Verification items for this drawing (mm, ordinates from the low corner). Round coordinates to 2 decimals unless told otherwise and drop trailing zeros. Order: outer loops, then holes, each group sorted by start corner. A loop starts at its lowest first (then second) coordinate and runs counter-clockwise, first axis right, second up. Notation, with made-up numbers: (85.5, -18) -> (129.5, -18) arc R33 ccw to (129.5, 17) -> close; hole circle Ø11 at (52.25, 16.5). An arc over 180 degrees is marked (long way). Put each result on its own line as item: value.
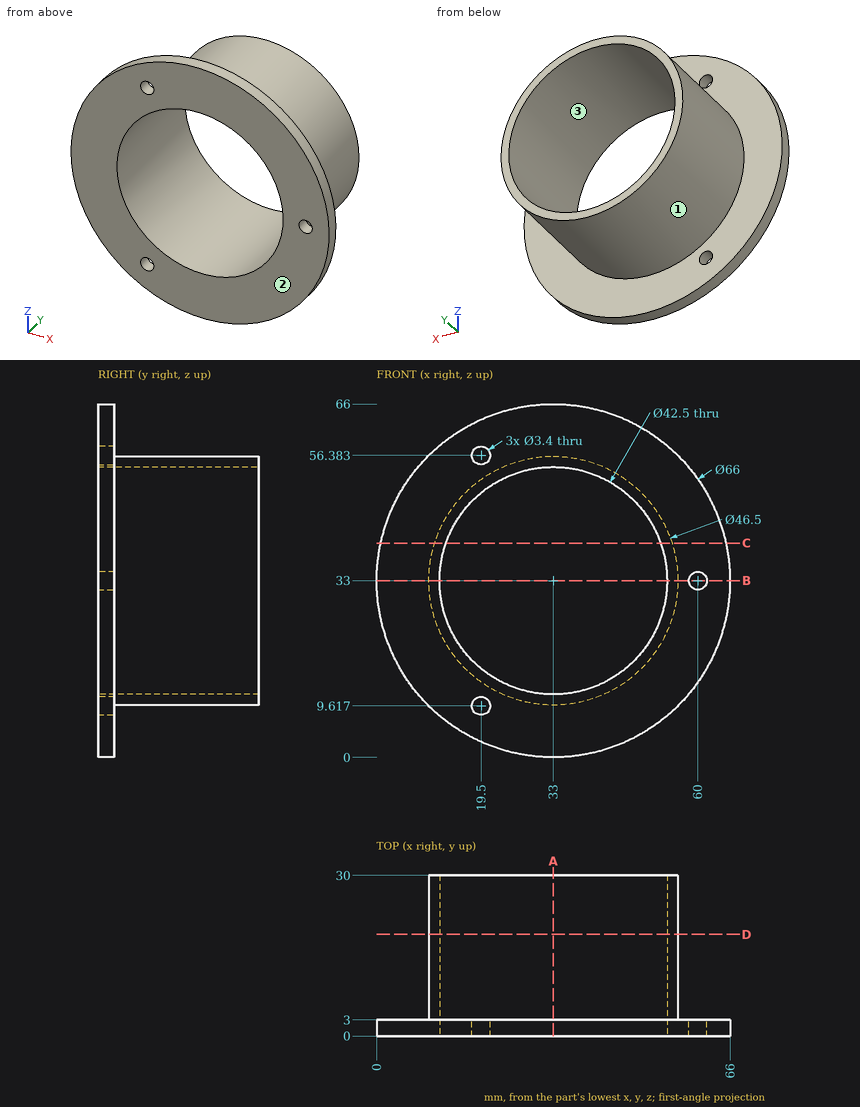
Item 1: Section check D-D on y = 19. Record the boundary of the cut face in (x, z).
Check sheet entries:
outline: circle Ø46.5 at (33, 33); hole circle Ø42.5 at (33, 33)
Item 2: Section check C-C on z = 40. Record the boundary of the cut face in (x, y), then the cut area to 3 significant figures.
Check sheet entries:
outline: (0.75, 0) -> (12.94, 0) -> (12.94, 30) -> (10.83, 30) -> (10.83, 3) -> (0.75, 3) -> close; (53.06, 0) -> (65.25, 0) -> (65.25, 3) -> (55.17, 3) -> (55.17, 30) -> (53.06, 30) -> close
area: 187 mm^2
Item 3: Section check B-B on z = 33. Record the boundary of the cut face in (x, y), then the cut area to 3 significant figures.
Check sheet entries:
outline: (0, 0) -> (11.75, 0) -> (11.75, 30) -> (9.75, 30) -> (9.75, 3) -> (0, 3) -> close; (54.25, 0) -> (58.3, 0) -> (58.3, 3) -> (56.25, 3) -> (56.25, 30) -> (54.25, 30) -> close; (61.7, 0) -> (66, 0) -> (66, 3) -> (61.7, 3) -> close
area: 168 mm^2
Item 4: Section check A-A on x = 33. Record the boundary of the cut face in (y, z).
Check sheet entries:
outline: (0, 0) -> (3, 0) -> (3, 9.75) -> (30, 9.75) -> (30, 11.75) -> (0, 11.75) -> close; (0, 54.25) -> (30, 54.25) -> (30, 56.25) -> (3, 56.25) -> (3, 66) -> (0, 66) -> close
Item 5: Release check for a two-part mould opening along Z. For the marked faces 1, 2 and 3 record: +Z half, -Z half, draft (parallel to the pull), parting line (faces both ways), or undercut.
Check sheet entries:
face 1: parting line
face 2: draft
face 3: undercut
Item 6: Material ranges on L1, parallel to X at y = 1.85, z = 33; L2, parallel to X at y = 15.75, z = 33; L3, parallel to Z at x = 40, y = 18.25 (1 decimal), recorded low to high. Write a range as [from, to].
Check sheet entries:
L1: x = [0, 11.75], [54.25, 58.3], [61.7, 66]
L2: x = [9.75, 11.75], [54.25, 56.25]
L3: z = [10.8, 12.9], [53.1, 55.2]
Item 7: Gauge pin test, flat ends, axial feed: pin 1 Ø1 at (x, y) = (8, 24) entering from +Z; pin 2 Ø8 at (y, z) = (13, 44.5) entering from +X; pin 3 Ø5.5 at (x, z) = (19.5, 56.38) entering from +Y; pin 4 Ø2 at (x, y) = (17, 22) entering from -Z (1 decimal). Record the tip position at first contact, or that the pin passes through.
Check sheet entries:
pin 1: passes through
pin 2: stops at x = 55.01
pin 3: stops at y = 3
pin 4: stops at z = 15.2
